The drawing under review shows one solid part. Ordinate dimensions are in mm from its lowest x, y, z. A direction names the side the tool comes from. Round coordinates to 2 decimals unless told otherwise and drop trailing zeros. Order: outer loops, then holes, each group sorted by start corner. A loop starts at its lowest first (then second) coordinate and runs counter-clockwise, first axis right, second up. Notation, with made-up numbers: M -18.75,68.5 L 32.25,68.5 A20 cw 32.25,92.5 Z; hole C 10.5,-28 d5. An arc over 180 degrees is marked long. Answer as a JSON object with one key per item and string values.
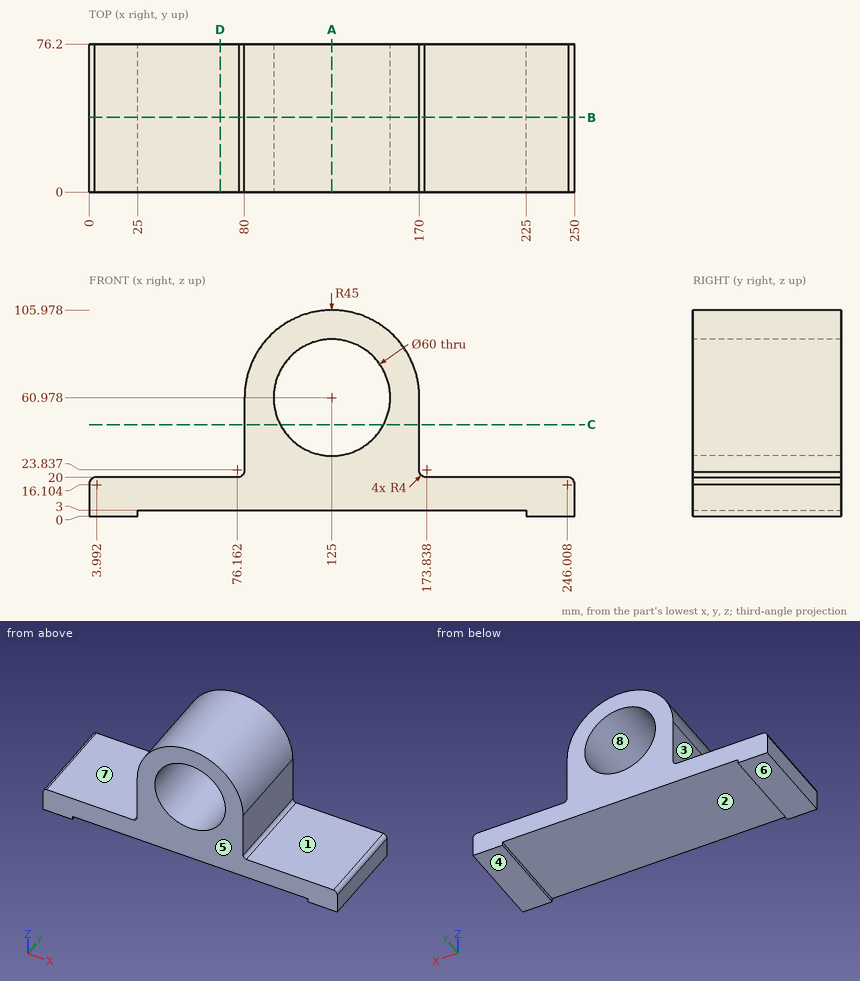
1) Add section B-B on y = 38.5. State the section outline as (x, z) points, and give its area (3 significant figures).
Geometry check:
{"outline": "M 0,0 L 25,0 L 25,3 L 225,3 L 225,0 L 250,0 L 250,16.36 A4 ccw 246.91,20 L 172.71,20 A4 cw 170,22.71 L 170,60.98 A45 ccw 80,60.98 L 80,22.71 A4 cw 77.29,20 L 3.09,20 A4 ccw 0,16.36 Z; hole C 125,60.98 d60", "area": "8,440 mm²"}
2) Mouldability with a two-part tool opening along Z and no side actions: class the marked faces 5, 6, 7 and 8 as +Z half, -Z half, draft (parallel to the pull), parting line (faces both ways), or undercut.
Geometry check:
{"face 5": "draft", "face 6": "-Z half", "face 7": "+Z half", "face 8": "undercut"}
3) Machinability: for the marked faces 1, 2, 3 and 4, which of the approach directions +Z, -Z, +X, -X, +Y, -Y give a long, thin tool a straight path to every point of the face, cutting with its end or side? Answer none if there is none.
Geometry check:
{"face 1": "+Z, +X, +Y, -Y", "face 2": "-Z, +Y, -Y", "face 3": "+Z, -X, +Y, -Y", "face 4": "-Z, +X, -X, +Y, -Y"}
4) Insertion check: P1, Ø3.5, axis at y = 50, z = 1.5, coming from the -X side; P2, Ø12, axis at y = 20, z = 23, coming from the -X side; P3, Ø19, axis at y = 49, z = 34.5, coming from the +X side; P4, Ø10, axis at x = 149.5, y = 10.5, coming from the +Z side (1 decimal). Each pin has a flat end and moves straight along its axis. Give the tip position at first contact, or say it passes through.
Geometry check:
{"P1": "stops at x = 0", "P2": "stops at x = 0.09", "P3": "stops at x = 170", "P4": "stops at z = 101.5"}
5) Add section C-C on z = 47. State the section outline as (x, y) points (1 decimal).
Geometry check:
{"outline": "M 80,0 L 98.5,0 L 98.5,76.2 L 80,76.2 Z; M 151.5,0 L 170,0 L 170,76.2 L 151.5,76.2 Z"}
6) Add section D-D on x = 67.5. State the section outline as (y, z) points.
Geometry check:
{"outline": "M 0,3 L 76.2,3 L 76.2,20 L 0,20 Z"}
7) For L1, parallel to Z at x = 125, y = 52.5; L2, parallel to Z at x = 176, y = 46; L3, parallel to X at y = 30.5, z = 47.5, list the stretches that pass through material, from the lowest coordinate up.
Geometry check:
{"L1": "z = 3 to 30.98, 90.98 to 105.98", "L2": "z = 3 to 20", "L3": "x = 80 to 98.2, 151.8 to 170"}
8) Add section A-A on x = 125. State the section outline as (y, z) points.
Geometry check:
{"outline": "M 0,3 L 76.2,3 L 76.2,30.98 L 0,30.98 Z; M 0,90.98 L 76.2,90.98 L 76.2,105.98 L 0,105.98 Z"}
